Model file for the job. Use its own axes, mm. Coordinates: 2 decimals unless noted, no trailing zeros. Order: outer loops, then holes, each group sorted by start corner. A loop starts at its lowest first (then second) coordinate and runs counter-clockwise, first axis right, second up. Notation, with made-up numbers: (26.25, 83.5) -> (62.25, 83.5) arc R20 ccw to (62.25, 99.5) -> close; hole circle Ø9 at (37, 76). An arc over 180 degrees is marked (long way). Use CSV: the item, a comma, the result in double quotes. Start each with the question number.
(1) Pull direction Y, two halves, no side cores. Call faces 1 (the flat face through (4, 14, 6)), 2 (the cylindrical face through (1.97, 21.65, -26.12)), 3 (the flat face through (1.97, 7.52, 28.72)), 4 (the cylindrical face through (1.972, 5.782, 11.924)): pulls with the +Y half, pulls with the -Y half, needs draft (parallel to the pull), parting line crosses it, or undercut.
(2) Cut at B-B on y = 26.75. Write the cut outline in (x, z), plus the area to 3 significant figures.
(3) Cut at A-A on x = 2.85. Write the cut outline in (y, z).
(4) Probe L1, parallel to Z at x = 1.4, y = 20.5; L2, parallel to Z at x = 3.2, y = 19.75; L3, parallel to Y at x = 2.4, z = 30.5. List the from-to ranges inside material, lowest first.
(5) Pin check, flat tips, straight feed: pin 1 Ø1.5 at (x, z) = (1, 26.5) entering from +Y; pin 2 Ø2 at (x, z) = (2.5, 2.5) entering from -Y; pin 3 Ø2 at (x, z) = (0.5, -4) entering from +Y. Stop position of each tip, or through.
(6) Cut at C-C on z = -21. Write the cut outline in (x, y), plus the area to 3 significant figures.
```python
from build123d import *

# Parameters (mm, degrees)
SKETCH_1_R      = 1.6
SKETCH_1_R_2    = 2.6
EXTRUDE_1_DEPTH = 4


with BuildPart() as part:
    # 草图1 → 凸台-拉伸1 (new body)
    with BuildSketch(Plane(origin=(0, 0, 0), x_dir=(0, 0, -1), z_dir=(1, 0, 0))):
        with BuildLine():
            Line((15.96147647, -1.109625561), (28.630049258, 11.041044095))
            Line((28.630049258, 11.041044095), (29.531620026, 24.009743728))
            Line((29.531620026, 24.009743728), (-32.319101296, 28.309542775))
            ThreePointArc((-32.319101296, 28.309542775), (-40.839313336, 22.108629409), (-36.779478782, 12.384274255))
            Line((-36.779478782, 12.384274255), (-20.433580884, 2.523050705))
            ThreePointArc((-20.433580884, 2.523050705), (-18.281565047, 1.550445439), (-15.96147647, 1.109625561))
            Line((-15.96147647, 1.109625561), (15.96147647, -1.109625561))
        make_face()
        with Locations((25.263844519, 20.296781)):
            Circle(SKETCH_1_R, mode=Mode.SUBTRACT)
        with Locations((-8.654292981, 22.654735317)):
            Circle(SKETCH_1_R, mode=Mode.SUBTRACT)
        with Locations((9.345707019, 10.376844831)):
            Circle(SKETCH_1_R, mode=Mode.SUBTRACT)
        with Locations((-10.654292981, 6.755156769)):
            Circle(SKETCH_1_R, mode=Mode.SUBTRACT)
        with Locations((-32.654292981, 19.816154374)):
            Circle(SKETCH_1_R_2, mode=Mode.SUBTRACT)
    extrude(amount=EXTRUDE_1_DEPTH)


solid = part.part
```
Outcome:
1,face 1,"needs draft"
1,face 2,"undercut"
1,face 3,"pulls with the -Y half"
1,face 4,"undercut"
2,outline,"(0, 9.89) -> (4, 9.89) -> (4, 37.57) -> (0, 37.57) -> close"
2,area,"111 mm2"
3,outline,"(-1.11, -15.96) -> (11.04, -28.63) -> (24.01, -29.53) -> (28.31, 32.32) arc R8.5 ccw to (12.38, 36.78) -> (2.52, 20.43) arc R10 ccw to (1.11, 15.96) -> close; hole circle Ø3.2 at (6.76, 10.65); hole circle Ø3.2 at (10.38, -9.35); hole circle Ø5.2 at (19.82, 32.65); hole circle Ø3.2 at (20.3, -25.26); hole circle Ø3.2 at (22.65, 8.65)"
4,L1,"-29.29 to -26.85, -23.68 to 30.15, 35.16 to 41.13"
4,L2,"-29.24 to -26.77, -23.76 to 30.06, 35.25 to 41.15"
4,L3,"8.6 to 18.36, 21.27 to 28.18"
5,pin 1,"y = 27.96"
5,pin 2,"y = 0.1"
5,pin 3,"y = 25.85"
6,outline,"(0, 3.72) -> (4, 3.72) -> (4, 24.6) -> (0, 24.6) -> close"
6,area,"83.5 mm2"
